Could you check a few things on this model? Use its own coordinates, in mm. A direction names the side the tool comes from. Give positions to 0.01 mm unless a question says otherwise; leave off trailing zeros. Order: outer loops, then holes, each group sorted by start corner. A loop starts at its lowest first (then second) coordinate and runs counter-clockwise, first axis right, second up. Notation, with made-up numbers: (-40, -3.75) -> (16, -3.75) arc R11 ccw to (16, 11.25) -> close; hole circle Ø10 at (26.5, 66.25). An arc over 180 degrees is marked (long way). One line per item, written item: value.
```python
from build123d import *

# Parameters (mm, degrees)
SKETCH1_W           = 53.6
SKETCH1_H           = 45.6
SKETCH1_W_2         = 23.6
SKETCH1_H_2         = 15.6
BOSS_EXTRUDE1_DEPTH = 6
SKETCH4_W           = 11
SKETCH4_H           = 5.8
SKETCH4_W_2         = 5.8
SKETCH4_H_2         = 11
CUT_EXTRUDE1_DEPTH  = 5
CUT_EXTRUDE2_DEPTH  = 5
SKETCH6_W           = 6.037335391
SKETCH6_H           = 12.047111719
CUT_EXTRUDE3_DEPTH  = 5
BOSS_EXTRUDE3_DEPTH = 1
SKETCH8_W           = 25
SKETCH8_H           = 17
CUT_EXTRUDE4_DEPTH  = 36.875897201


with BuildPart() as part:
    # Sketch1 → Boss-Extrude1 (new body)
    with BuildSketch(Plane(origin=(0, 0, 0), x_dir=(1, 0, 0), z_dir=(0, 1, 0))):
        Rectangle(SKETCH1_W, SKETCH1_H)
        Rectangle(SKETCH1_W_2, SKETCH1_H_2, mode=Mode.SUBTRACT)
    extrude(amount=BOSS_EXTRUDE1_DEPTH)

    # Sketch4 → Cut-Extrude1 (cut)
    with BuildSketch(Plane.XZ):
        with Locations((-17.3, 0)):
            Rectangle(SKETCH4_W, SKETCH4_H)
        with Locations((0, -13.3)):
            Rectangle(SKETCH4_W_2, SKETCH4_H_2)
        with Locations((0, 13.3)):
            Rectangle(SKETCH4_W_2, SKETCH4_H_2)
        with Locations((17.3, 0)):
            Rectangle(SKETCH4_W, SKETCH4_H)
    extrude(amount=-CUT_EXTRUDE1_DEPTH, mode=Mode.SUBTRACT)

    # Sketch5 → Cut-Extrude2 (cut)
    with BuildSketch(Plane.XZ):
        Polygon((-2.9, -18.8), (-22.8, -18.8), (-22.8, -2.9), (-17.8, -2.9), (-17.8, -13.8), (-2.9, -13.8), align=None)
        Polygon((-2.9, 18.8), (-2.9, 13.8), (-17.8, 13.8), (-17.8, 2.9), (-22.8, 2.9), (-22.8, 18.8), align=None)
        Polygon((22.8, -18.8), (22.8, -2.9), (17.8, -2.9), (17.8, -13.8), (2.9, -13.8), (2.9, -18.8), align=None)
        Polygon((2.9, 18.8), (2.9, 13.8), (17.8, 13.8), (17.8, 2.9), (22.8, 2.9), (22.8, 18.8), align=None)
    extrude(amount=-CUT_EXTRUDE2_DEPTH, mode=Mode.SUBTRACT)

    # Sketch6 → Cut-Extrude3 (cut)
    with BuildSketch(Plane.XZ):
        with Locations((-25.818667696, -12.776444141)):
            Rectangle(SKETCH6_W, SKETCH6_H)
    extrude(amount=-CUT_EXTRUDE3_DEPTH, mode=Mode.SUBTRACT)

    # Sketch7 → Boss-Extrude3 (add)
    with BuildSketch(Plane.XZ):
        Polygon((22.8, -18.8), (-26.8, -18.8), (-26.8, -22.8), (26.8, -22.8), (26.8, 22.8), (-26.8, 22.8), (-26.8, -6.752888281), (-22.8, -6.752888281), (-22.8, 18.8), (22.8, 18.8), align=None)
        Polygon((-17.8, -2.9), (-17.8, -13.8), (-2.9, -13.8), (-2.9, -7.8), (-11.8, -7.8), (-11.8, -2.9), align=None)
        Polygon((-2.9, 13.8), (-17.8, 13.8), (-17.8, 2.9), (-11.8, 2.9), (-11.8, 7.8), (-2.9, 7.8), align=None)
        Polygon((2.9, -13.8), (17.8, -13.8), (17.8, -2.9), (11.8, -2.9), (11.8, -7.8), (2.9, -7.8), align=None)
        Polygon((17.8, 2.9), (17.8, 13.8), (2.9, 13.8), (2.9, 7.8), (11.8, 7.8), (11.8, 2.9), align=None)
    extrude(amount=BOSS_EXTRUDE3_DEPTH)

    # Sketch8 → Cut-Extrude4 (cut, through all)
    with BuildSketch(Plane(origin=(0, 6, 0), x_dir=(1, 0, 0), z_dir=(0, 1, 0))):
        Rectangle(SKETCH8_W, SKETCH8_H)
    extrude(amount=-CUT_EXTRUDE4_DEPTH, mode=Mode.SUBTRACT)


solid = part.part
```
1) Suppose I cut it at A-A, the plane x = -1. Write out the boundary of the cut face in (y, z), then the cut area to 3 significant figures.
Answer below:
outline: (-1, -22.8) -> (6, -22.8) -> (6, -8.5) -> (5, -8.5) -> (5, -18.8) -> (-1, -18.8) -> close; (-1, 18.8) -> (5, 18.8) -> (5, 8.5) -> (6, 8.5) -> (6, 22.8) -> (-1, 22.8) -> close
area: 76.6 mm2
2) Suppose I cut it at C-C, the plane y = 4. State how many separate pieces and enclosed holes the cut face has, then the cut area to 3 significant figures.
Answer below:
separate pieces: 5
enclosed holes: 0
area: 1,120 mm2
3) We'd pull the mould along X, two halves only. Please class faces 4 (the flat face through (15, 2, -2.9)), 5 (the flat face through (26.8, 3, 0)), 6 (the flat face through (-2, 2, -18.8)): +X half, -X half, draft (parallel to the pull), parting line (faces both ways), or undercut.
Answer below:
face 4: undercut
face 5: +X half
face 6: draft
4) Suppose I cut it at B-B, the plane z = 6. Write out the boundary of the cut face in (x, y), then the cut area to 3 significant figures.
Answer below:
outline: (-26.8, -1) -> (-22.8, -1) -> (-22.8, 5) -> (-17.8, 5) -> (-17.8, -1) -> (-12.5, -1) -> (-12.5, 6) -> (-26.8, 6) -> close; (12.5, -1) -> (17.8, -1) -> (17.8, 5) -> (22.8, 5) -> (22.8, -1) -> (26.8, -1) -> (26.8, 6) -> (12.5, 6) -> close
area: 140 mm2
5) Suppose I cut it at D-D, the plane x = 22. Write out the boundary of the cut face in (y, z).
Answer below:
outline: (-1, -22.8) -> (6, -22.8) -> (6, 22.8) -> (-1, 22.8) -> (-1, 18.8) -> (5, 18.8) -> (5, -18.8) -> (-1, -18.8) -> close
6) If I drill on line 1 along Z through (x, y) = (-11.5, 2); line 2 along Z through (x, y) = (-15, 1.5); line 3 along X through (y, z) = (4.25, 4.5), over which ranges is the centre line in solid material (lowest first)?
Answer below:
line 1: z = -22.8 to -18.8, -13.8 to -8.5, 8.5 to 13.8, 18.8 to 22.8
line 2: z = -22.8 to -18.8, -13.8 to -2.9, 2.9 to 13.8, 18.8 to 22.8
line 3: x = -26.8 to -22.8, -17.8 to -12.5, 12.5 to 17.8, 22.8 to 26.8
7) For faces 1 (the flat face through (10, 2, -13.8)), 2 (the flat face through (-0.2, 5.7, 8.5)), 3 (the flat face through (-10, 2, 13.8)), which set-ups out of +Z, -Z, +X, -X, +Y, -Y let a thin tool reach every point of the face, with its end or its side?
Answer below:
face 1: -X, -Y
face 2: +Y, -Y
face 3: -Y
